Work out the finished part from the listing and answer in its coordinate system (mm). A direction names the side the tool comes from. Coordinates: 2 decimals unless noted, no trailing zeros. Order: outer loops, then holes, each group sorted by start corner. A loop starts at its lowest first (then second) coordinate and runs counter-clockwise, first axis right, second up. Notation, with made-up numbers: M -2,-37 L 21,-37 A38 ccw 21,1 Z; hole C -23,15 d10. An arc over 180 degrees is marked long. Write item = value, one per line. Start each with the question number.
Q1. Determine the mould class of faces 5 (the flat face through (3.931, -21.693, 6.493)), 6 (the flat face through (-20.752, 7.442, 6.493)) for opening direction Y: released by +Y, released by -Y, zero draft, split by the parting line, or undercut.
Q2. Find section B-B on z = 2.75. Give the vertices of the cut face in (x, y), and give its area (3 significant figures).
Q3. Find section A-A on y = -13. Give the vertices of the cut face in (x, z), and give its area (3 significant figures).
Q4. Straight lines are drawn through the part: line 1 along Y through (x, z) = (19, 5.75); line 2 along Y through (x, z) = (-7, 4.75); line 3 along X through (y, z) = (-16.5, 5.25). For each, find the intervals that lie inside material, in ascending order.
Q5. Each of these flat-tipped pins is pushed along its axis until it touches: P1, Ø2, axis at y = 19, z = 4, coming from the -X side; P2, Ø18, axis at x = -22.52, y = -13, coming from the -Z side; P3, Ø1.5, axis at y = -1, z = 1.5, coming from the -X side; P4, Ø1, axis at y = 32.5, z = 2, coming from the +X side. Where does it stop, or does it pass through?
Q6. A tool of negligible diameter and unlimited length cuts with its end or side. For faces 1 (the flat face through (-17, 14.744, 4)), 2 (the flat face through (21.36, 7.51, 3.54)), 3 (the flat face through (-4.03, -21.521, 0.507)), 4 (the cylindrical face through (0.015, -28.488, 3.465)), from which of +Z, -Z, +X, -X, +Y, -Y can it reach the whole face along a straight path? Write none if from no direction.
Q7. Find section C-C on y = 26. Give the vertices of the cut face in (x, z), and give its area (3 significant figures).
```python
from build123d import *

# Parameters (mm, degrees)
F0_R            = 11.1
F1_DEPTH        = 7
F2_COUNT        = 3
F5_DEPTH        = 7
F5_COPIES_COUNT = 3
F6_D            = 5
F6_COPIES_COUNT = 3
F7_R            = 1
F8_SIZE         = 0.99999


# Not quite as in the source:
# - a fillet or chamfer is up to 0.001 mm smaller than in the source, because OpenCascade refuses the exact size
# - a pattern or mirror of a feature is missing from the dataset's text; its kind, count and spacing are read off the source's solid


with BuildPart() as f1:
    # F0 (on Top) → F1 (new body)
    with BuildSketch(Plane.XY):
        with BuildLine():
            ThreePointArc((-9.612881982, 5.55), (0, 11.1), (9.612881982, 5.55))
            Line((9.612881982, 5.55), (11.2583302492, 6.5))
            Line((11.2583302492, 6.5), (12.2109581934, 7.05))
            ThreePointArc((12.2109581934, 7.05), (10.6166604984, 13), (12.2109581934, 18.95))
            ThreePointArc((12.2109581934, 18.95), (0, 40.1), (-12.2109581934, 18.95))
            ThreePointArc((-12.2109581934, 18.95), (-10.6166604984, 13), (-12.2109581934, 7.05))
            Line((-12.2109581934, 7.05), (-11.2583302492, 6.5))
            Line((-11.2583302492, 6.5), (-9.612881982, 5.55))
        make_face()
        with Locations((0, 26)):
            Circle(F0_R, mode=Mode.SUBTRACT)
    extrude(amount=F1_DEPTH)

    # F2: F1 ×3 about axis
    f2_axis = Axis((0, 0, 0), (0, 0, 1))


with BuildPart() as f1_1:
    add(f1.part)
    for i in range(1, F2_COUNT):
        add(f1.part.rotate(f2_axis, i * 360 / F2_COUNT))

    # F4 (on face) → F5 (join)
    with BuildSketch(Plane.XY.offset(7)):
        with BuildLine():
            ThreePointArc((-18.1411493779, 1.9336138494), (-12.2109581934, 7.05), (-10.7451334036, 14.7438892904))
            Line((-10.7451334036, 14.7438892904), (-25.5371653521, 14.7438892904))
            Line((-25.5371653521, 14.7438892904), (-18.1411493779, 1.9336138494))
        make_face()
    f5 = extrude(amount=-F5_DEPTH)

    # F5_copies: F5 ×3 about axis
    f5_copies_axis = Axis((0, 0, 0), (0, 0, 1))
    for i in range(1, F5_COPIES_COUNT):
        add(f5.rotate(f5_copies_axis, i * 360 / F5_COPIES_COUNT))

    # F6 (through all)
    with Locations(Plane.XY.offset(7)):
        with Locations((-15.8686004579, 9.161740746)):
            f6 = Hole(F6_D / 2)

    # F6_copies: F6 ×3 about axis
    f6_copies_axis = Axis((0, 0, 0), (0, 0, 1))
    for i in range(1, F6_COPIES_COUNT):
        add(f6.rotate(f6_copies_axis, i * 360 / F6_COPIES_COUNT), mode=Mode.SUBTRACT)

    # F7
    f7_edges = [f1_1.edges().sort_by_distance(p)[0] for p in [
        (-25.537165, 14.743889, 3.5),
        (25.537165, 14.743889, 3.5),
        (0, -29.487779, 3.5),
    ]]
    fillet(f7_edges, radius=F7_R)

    # F8 (size 1 in the source; OpenCascade refuses exactly that, so slightly less here)
    f8_edges = [f1_1.edges().sort_by_distance(p)[0] for p in [
        (17.275124, 14.743889, 0),
        (24.67114, 14.243889, 0),
        (11.279496, 16.916139, 0),
        (21.406145, 7.588752, 0),
        (0, 40.1, 0),
        (20.289554, 1.310261, 0),
        (-11.279496, 16.916139, 0),
        (34.727619, -20.05, 0),
        (-17.275124, 14.743889, 0),
        (9.010058, -18.2264, 0),
        (-24.67114, 14.243889, 0),
        (4.131021, -22.332641, 0),
        (-21.406145, 7.588752, 0),
        (0, -28.487779, 0),
        (-20.289554, 1.310261, 0),
        (-4.131021, -22.332641, 0),
        (-34.727619, -20.05, 0),
        (-9.010058, -18.2264, 0),
        (-16.96666, -22.612882, 0),
        (1.25, -20.488545, 0),
        (28.06666, -3.387118, 0),
        (-9.612882, -5.55, 0),
        (-18.3686, 9.161741, 0),
        (17.1186, 11.326804, 0),
        (-11.1, 26, 0),
        (17.275124, 14.743889, 7),
        (24.67114, 14.243889, 7),
        (11.279496, 16.916139, 7),
        (21.406145, 7.588752, 7),
        (0, 40.1, 7),
        (20.289554, 1.310261, 7),
        (-11.279496, 16.916139, 7),
        (34.727619, -20.05, 7),
        (-17.275124, 14.743889, 7),
        (9.010058, -18.2264, 7),
        (-24.67114, 14.243889, 7),
        (4.131021, -22.332641, 7),
        (-21.406145, 7.588752, 7),
        (0, -28.487779, 7),
        (-20.289554, 1.310261, 7),
        (-4.131021, -22.332641, 7),
        (-34.727619, -20.05, 7),
        (-9.010058, -18.2264, 7),
        (-16.96666, -22.612882, 7),
        (1.25, -20.488545, 7),
        (28.06666, -3.387118, 7),
        (-9.612882, -5.55, 7),
        (-18.3686, 9.161741, 7),
        (17.1186, 11.326804, 7),
        (-11.1, 26, 7),
    ]]
    chamfer(f8_edges, length=F8_SIZE)


solid = f1_1.part
```
Findings below:
q1.face_5 = released by -Y
q1.face_6 = undercut
q2.outline = M -24.67,13.24 L -18.14,1.93 A11.9 cw -22.52,1.1 A14.1 ccw long -10.31,-20.05 A11.9 cw -7.4,-16.68 L -0.87,-27.99 A1 ccw 0.87,-27.99 L 7.4,-16.68 A11.9 cw 10.31,-20.05 A14.1 ccw long 22.52,1.1 A11.9 cw 18.14,1.93 L 24.67,13.24 A1 ccw 23.81,14.74 L 10.75,14.74 A11.9 cw 12.21,18.95 A14.1 ccw long -12.21,18.95 A11.9 cw -10.75,14.74 L -23.81,14.74 A1 ccw Z; hole C -22.52,-13 d22.2; hole C -15.87,9.16 d5; hole C 0,0 d22.2; hole C 0,26 d22.2; hole C 0,-18.32 d5; hole C 22.52,-13 d22.2; hole C 15.87,9.16 d5
q2.area = 1,310 mm^2
q3.outline = M -36.62,1 L -35.62,0 L -34.62,0 L -33.62,1 L -33.62,6 L -34.62,7 L -35.62,7 L -36.62,6 Z; M -11.42,1 L -10.42,0 L 10.42,0 L 11.42,1 L 11.42,6 L 10.42,7 L -10.42,7 L -11.42,6 Z; M 33.62,1 L 34.62,0 L 35.62,0 L 36.62,1 L 36.62,6 L 35.62,7 L 34.62,7 L 33.62,6 Z
q3.area = 196 mm^2
q4.line_1 = -26.65 to -23.53, -2.47 to 1.63, 3.42 to 14.74
q4.line_2 = -17.36 to -8.61, 8.61 to 17.39, 34.61 to 38.24
q4.line_3 = -36.18 to -33.05, -11.98 to -1.71, 1.71 to 11.98, 33.05 to 36.18
q5.P1 = -12.76
q5.P2 = through
q5.P3 = -31.02
q5.P4 = 12.76
q6.face_1 = +Z, -Z, -X
q6.face_2 = +Z, -Z, +X
q6.face_3 = -Z, -Y
q6.face_4 = +Z, -Z, -Y
q7.outline = M -14.1,1 L -13.1,0 L -12.1,0 L -11.1,1 L -11.1,6 L -12.1,7 L -13.1,7 L -14.1,6 Z; M 11.1,1 L 12.1,0 L 13.1,0 L 14.1,1 L 14.1,6 L 13.1,7 L 12.1,7 L 11.1,6 Z
q7.area = 38.0 mm^2
